Can you work these out from the model? Positions are in its coordinate system, mm. Face numbers are marked on the shaded views. A direction names the side the tool comes from. Coordinates: 2 decimals unless noted, no trailing zeros. Order: outer loops, then holes, each group sorted by start corner. A loop starts at its lowest first (then second) coordinate and runs counter-clockwise, first axis right, second up. Notation, with made-up numbers: (12, -33.5) - (61, -33.5) arc R16 cw to (61, -2.5) - close; hole circle Ø5 at (48.25, 69.25). An arc over 180 degrees is marked (long way). Use a Markdown table: item, result. Add a question column.
(1) If I drill on L1, parallel to X at y = -7, z = 3.75; L2, parallel to X at y = -10.5, z = 3.25; L3, parallel to Z at x = 6.5, y = -5.5, over which ranges is the centre line in solid material (lowest first)? Write a range as [from, to].
(2) I want a section at C-C (y = -4.5). List the corners of the cut face in (x, z) for me.
(3) I want a section at D-D (y = -1.25). List the corners of the cut face in (x, z) for me, and give its area (3 significant figures).
(4) For pin 1 Ø5.5 at (x, z) = (0, -3.5) entering from +Y; pin 2 Ø2 at (x, z) = (-6.5, 13.5) entering from -Y; pin 3 Ø5 at (y, z) = (-10.5, 14.5) entering from -X, each with a flat end and sliding along its axis, tell me the tip position at first contact or that it passes through.
(5) I want a section at B-B (x = 1.75). List the corners of the cut face in (y, z) for me, and give its area (3 significant figures).
(6) We'd pull the mould along X, two halves only. Please class the marked faces 1, 2, 3 and 4: pulls with the +X half, pulls with the -X half, needs draft (parallel to the pull), parting line crosses it, or undercut.
(7) On a 3-axis mill with a long thin cutter (end or side, diameter ignored), from which of +Z, -Z, +X, -X, +Y, -Y can I reach the whole of each face in a straight line? I mean the marked faces 5, 6, 7 and 8. Say none if no direction works.
(8) I want a section at A-A (z = 6.5). List the corners of the cut face in (x, y) for me, and give its area (3 significant figures).
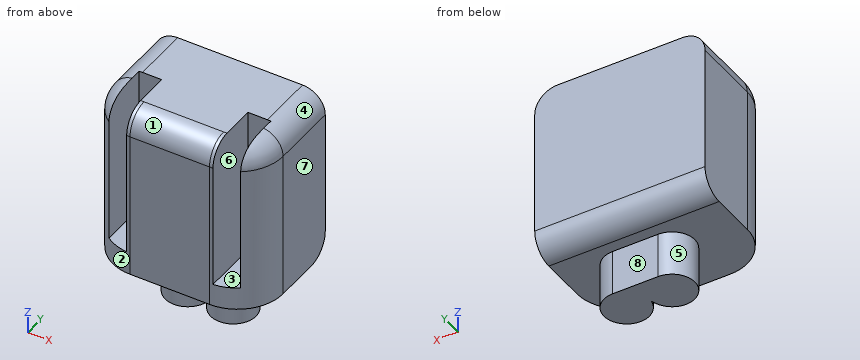
```python
from build123d import *

# Parameters (mm, degrees)
F0_W        = 19.05
F0_H        = 19.05
F1_DEPTH    = 12.7
F2_R        = 2.54
F3_T1_DEPTH = 31.75
F3_T4_ANGLE = 90
F3_T6_ANGLE = 90
F5_W        = 2.54
F5_H        = 16.51
F6_DEPTH    = 6.35
F7_R        = 2.54
F9_DEPTH    = 5.08


# Not quite as in the source:
# - a fillet or chamfer that OpenCascade refuses, or shapes differently, is made with other operations: its cross-section is extruded or revolved along the edge and cut away or added


with BuildPart() as f1:
    # F0 (on Front) → F1 (new body)
    with BuildSketch(Plane.XZ):
        with Locations((0.0981341409, 9.525)):
            Rectangle(F0_W, F0_H)
    extrude(amount=F1_DEPTH)

    # F2
    f2_edges = [f1.edges().sort_by_distance(p)[0] for p in [
        (9.623134, -6.35, 19.05),
        (-9.426866, -6.35, 19.05),
        (0.098134, -12.7, 19.05),
    ]]
    fillet(f2_edges, radius=F2_R)

    # F3: fillet of radius 5.08 on 2 edges, made by hand

    # F3_s2 → F3_t1 (cut)
    with BuildSketch(Plane.XY.offset(-12.7)):
        with BuildLine():
            ThreePointArc((9.6231341409, -7.62), (8.1352365894, -11.2121024484), (4.5431341409, -12.7))
            Line((4.5431341409, -12.7), (9.6231341409, -12.7))
            Line((9.6231341409, -12.7), (9.6231341409, -7.62))
        make_face()
        with BuildLine():
            ThreePointArc((-9.4268658591, -7.62), (-7.9389683075, -11.2121024484), (-4.3468658591, -12.7))
            Line((-4.3468658591, -12.7), (-9.4268658591, -12.7))
            Line((-9.4268658591, -12.7), (-9.4268658591, -7.62))
        make_face()
    extrude(amount=F3_T1_DEPTH, mode=Mode.SUBTRACT)

    # F3_s3 → F3_t4 (revolve, cut)
    with BuildSketch(Plane.XZ.offset(7.62)):
        with BuildLine():
            ThreePointArc((-6.8868658591, 19.05), (-8.6829170833, 18.3060512242), (-9.4268658591, 16.51))
            Line((-9.4268658591, 16.51), (-9.4268658591, 19.05))
            Line((-9.4268658591, 19.05), (-6.8868658591, 19.05))
        make_face()
    revolve(axis=Axis((-4.3468658591, -7.62, 19.05), (0, 0, 1)), revolution_arc=F3_T4_ANGLE, mode=Mode.SUBTRACT)

    # F3_s5 → F3_t6 (revolve, cut)
    with BuildSketch(Plane.YZ.offset(4.5431341409)):
        with BuildLine():
            ThreePointArc((-10.16, 19.05), (-11.9560512242, 18.3060512242), (-12.7, 16.51))
            Line((-12.7, 16.51), (-12.7, 19.05))
            Line((-12.7, 19.05), (-10.16, 19.05))
        make_face()
    revolve(axis=Axis((4.5431341409, -7.62, 19.05), (0, 0, 1)), revolution_arc=F3_T6_ANGLE, mode=Mode.SUBTRACT)

    # F5 (on offset) → F6 (cut)
    with BuildSketch(Plane.XZ.offset(12.7)):
        with Locations((-5.9978658591, 10.795)):
            Rectangle(F5_W, F5_H)
        with Locations((6.1941341409, 10.795)):
            Rectangle(F5_W, F5_H)
    extrude(amount=-F6_DEPTH, mode=Mode.SUBTRACT)

    # F7
    f7_edges = [f1.edges().sort_by_distance(p)[0] for p in [
        (0.098134, 0, 0),
    ]]
    fillet(f7_edges, radius=F7_R)

    # F8 (on face) → F9 (join)
    with BuildSketch(Plane(origin=(0, 0, 0), x_dir=(1, 0, 0), z_dir=(0, 0, -1))):
        with BuildLine():
            ThreePointArc((0.7668002065, 6.7621773998), (0.7035904263, 6.8367161594), (0.6666799214, 6.927209903))
            ThreePointArc((0.6666799214, 6.927209903), (-3.7965534166, 7.9288424314), (-1.8068658591, 3.81))
            Line((-1.8068658591, 3.81), (3.2731341493, 3.81))
            ThreePointArc((3.2731341493, 3.81), (5.2094361027, 7.9938779495), (0.7668002065, 6.7621773998))
        make_face()
    extrude(amount=F9_DEPTH)


solid = f1.part
```
Answers follow:
| question | item | result |
|---|---|---|
| 1 | L1 | x = [-9.43, -7.27], [-4.73, 4.92], [7.46, 9.62] |
| 1 | L2 | x = [-8.53, -7.27], [-4.73, 4.92], [7.46, 8.73] |
| 1 | L3 | z = [0, 19.05] |
| 2 | outline | (-9.43, 0) - (-3.55, 0) - (-3.55, -5.08) - (5.01, -5.08) - (5.01, 0) - (9.62, 0) - (9.62, 16.51) arc R2.54 ccw to (7.08, 19.05) - (-6.89, 19.05) arc R2.54 ccw to (-9.43, 16.51) - close |
| 3 | outline | (-9.43, 0.35) - (9.62, 0.35) - (9.62, 16.51) arc R2.54 ccw to (7.08, 19.05) - (-6.89, 19.05) arc R2.54 ccw to (-9.43, 16.51) - close |
| 3 | area | 353 mm² |
| 4 | pin 1 | stops at y = -3.81 |
| 4 | pin 2 | stops at y = -11.78 |
| 4 | pin 3 | stops at x = -9.41 |
| 5 | outline | (-12.7, 0) - (-8.38, 0) - (-8.38, -5.08) - (-3.81, -5.08) - (-3.81, 0) - (-2.54, 0) arc R2.54 ccw to (0, 2.54) - (0, 19.05) - (-10.16, 19.05) arc R2.54 ccw to (-12.7, 16.51) - close |
| 5 | area | 262 mm² |
| 6 | face 1 | needs draft |
| 6 | face 2 | pulls with the -X half |
| 6 | face 3 | undercut |
| 6 | face 4 | pulls with the +X half |
| 7 | face 5 | -Z |
| 7 | face 6 | +Z, -Y |
| 7 | face 7 | +Z, -Z, +X, +Y, -Y |
| 7 | face 8 | -Z, +X, -X, +Y |
| 8 | outline | (-9.43, -7.62) arc R5.08 ccw to (-7.27, -11.78) - (-7.27, -6.35) - (-4.73, -6.35) - (-4.73, -12.69) arc R5.08 ccw to (-4.35, -12.7) - (4.54, -12.7) arc R5.08 ccw to (4.92, -12.69) - (4.92, -6.35) - (7.46, -6.35) - (7.46, -11.78) arc R5.08 ccw to (9.62, -7.62) - (9.62, 0) - (-9.43, 0) - close |
| 8 | area | 200 mm² |
